Part model, mm, in its own coordinate system. Face numbers are marked on the shaded views. A direction names the side the tool comes from. Give positions to 0.01 mm unless a question says otherwise; leave off trailing zeros. Write each loop counter-clockwise with the first axis right and the second up, starting at its lowest first coordinate (ties: lowest second). Pieces come first, ordered by that corner, then holes.
Autodesk Inventor part; units mm, degrees
ref_plane "Work Plane2" through (2.8, 0, 0) normal (0, 1, 0) x (1, 0, 0)
ref_plane "YZ Plane" through (0, 0, 0) normal (1, 0, 0) x (0, 1, 0)
ref_plane "XZ Plane" through (0, 0, 0) normal (0, 1, 0) x (-1, 0, 0)
sketch "Sketch1" plane through (0, 0, 0) normal (0, 0, 1) x (1, 0, 0)
  line L0 (5.7, 0) -> (45, 0)
  line L1 (45, 0) -> (45, 4.75)
  line L2 (45, 4.75) -> (5.25, 4.75)
  line L3 (0.85, 9.15) -> (0, 9.15)
  line L4 (-9, 0) -> (54, 0)
  line L5 (0, -1.83) -> (0, 10.98)
  line L6 (0, 5) -> (4.1386, 2.9366)
  line L7 (4.1386, 2.9366) -> (5.7, 0)
  line L8 (5.25, 4.75) -> (0.85, 9.15)
  line L9 (0, 9.15) -> (0, 5)
  dimension "d2" = 9.5
  dimension "d3" = 18.3
  dimension "d4" = 5.7
  dimension "d5" = 10
  dimension "d6" = 26.5
  dimension "d7" = 62
  dimension "d13" = 45
  dimension "d14" = 5.25
  dimension "d15" = 45
revolve "Body" add sketch "Sketch1" angle 360 about axis through (5.7, 0, 0) along (1, 0, 0) contours L7 L6 L5 L3 L8 L2 L1 L0
sketch "Sketch2" plane through (0, 0, 0) normal (-1, 0, 0) x (0, 0, 1)
  line L0 (0, -12.81) -> (0, 12.81)
  line L1 (-12.81, 0) -> (12.81, 0)
  line L2 (0, 5) -> (0, 0) construction
  line L3 (0, 0) -> (5, 0) construction
  arc A0 (1.5, 0) -> (0, 1.5) centre (0, 0) ccw construction
  line L4 (0, 0) -> (6.47, 6.47) construction
  arc A1 (1.75, 0) -> (0, 1.75) centre (0, 0) ccw construction
  line L5 (0.595, 4.9645) -> (0.8448, 1.5326)
  line L6 (4.9645, 0.595) -> (1.5326, 0.8448)
  arc A2 (0.8448, 1.5326) -> (1.5326, 0.8448) centre (1.5866, 1.5866) ccw
  arc A3 (5, 0) -> (4.9645, 0.595) centre (0, 0) ccw
  arc A4 (0.595, 4.9645) -> (0, 5) centre (0, 0) ccw
  arc A5 (4.9645, 0.595) -> (0.595, 4.9645) centre (0, 0) ccw
  line L7 (0.595, -4.9645) -> (0.8448, -1.5326)
  line L8 (4.9645, -0.595) -> (1.5326, -0.8448)
  arc A6 (1.5326, -0.8448) -> (0.8448, -1.5326) centre (1.5866, -1.5866) ccw
  arc A7 (4.9645, -0.595) -> (5, 0) centre (0, 0) ccw
  arc A8 (0, -5) -> (0.595, -4.9645) centre (0, 0) ccw
  arc A9 (0.595, -4.9645) -> (4.9645, -0.595) centre (0, 0) ccw
  line L9 (-0.595, 4.9645) -> (-0.8448, 1.5326)
  line L10 (-4.9645, 0.595) -> (-1.5326, 0.8448)
  arc A10 (-1.5326, 0.8448) -> (-0.8448, 1.5326) centre (-1.5866, 1.5866) ccw
  arc A11 (-4.9645, 0.595) -> (-5, 0) centre (0, 0) ccw
  arc A12 (0, 5) -> (-0.595, 4.9645) centre (0, 0) ccw
  arc A13 (-0.595, 4.9645) -> (-4.9645, 0.595) centre (0, 0) ccw
  arc A14 (-4.9645, -0.595) -> (-0.595, -4.9645) centre (0, 0) ccw
  arc A15 (-0.595, -4.9645) -> (0, -5) centre (0, 0) ccw
  arc A16 (-5, 0) -> (-4.9645, -0.595) centre (0, 0) ccw
  line L11 (-4.9645, -0.595) -> (-1.5326, -0.8448)
  arc A17 (-0.8448, -1.5326) -> (-1.5326, -0.8448) centre (-1.5866, -1.5866) ccw
  line L12 (-0.595, -4.9645) -> (-0.8448, -1.5326)
  circle A18 centre (0, 0) radius 9.15
  circle A19 centre (0, 0) radius 5
  dimension "d18" = 45
  dimension "d19" = 3
  dimension "d20" = 3.5
  dimension "d21" = 10
  dimension "d22" = 0.595
extrude "Slot" add sketch "Sketch2" against normal up to next draft 1 contours L7 A6 L8 A9 | A14 L11 A17 L12 | A13 L9 A10 L10 | L6 A2 L5 A5
fillet "Fillet1" radius 0.238 4 edges at (0, 5, 0) (0, 0, 5) (0, -5, 0) (0, 0, -5)
thread "Thread"
chamfer "Chamfer1" distance 1.03 distance2 4.2 1 edges at (45, -4.75, 0) measured on face at (45, -1.1851, 1.0499)
ref_plane "Work Plane2" through (2.8, 0, 0) normal (0, 1, 0) x (1, 0, 0)
equation "\"d2\" = NND"
equation "\"d3\" = KOD"
equation "\"d4\" = STI"
equation "\"d5\" = SDM"
equation "\"d13\" = 0.5 * SEWI"
equation "\"d14\" = KOH"
equation "\"d15\" = NLG"
equation "\"d19\" = 0.3 * SDM"
equation "\"d20\" = 0.35 * SDM"
equation "\"d21\" = SDM"
equation "\"d22\" = 0.5 * SBR"
equation "\"d45\" = STI"
equation "\"d25\" = 0.2 * SBR"
equation "\"d9\" = GEL"
equation "\"d11\" = -0.5 * GD2 + 0.5 * NND"
equation "\"d12\" = SPTZ"
equation "\"NND\" = 9.5"
equation "\"NLG\" = 45"
equation "\"GEL\" = 39.75"
equation "\"KOD\" = 18.3"
equation "\"KOH\" = 5.25"
equation "\"SDM\" = 10"
equation "\"STI\" = 5.7"
equation "\"SBR\" = 1.19"
equation "\"SPTZ\" = 4.2"
equation "\"GD2\" = 7.44"
equation "\"SEWI\" = 90deg"
equation "\"d0\" = NLG"
equation "\"d1\" = KOH"
equation "\"THREADDIA\" = 9.5"
equation "\"TOA\" = 30deg"
equation "\"PTC\" = 2.1"
equation "\"GD1\" = 7.85"
properties part number "ISO 7050 - ST 9.5 x 45 - F - H" material "Steel"
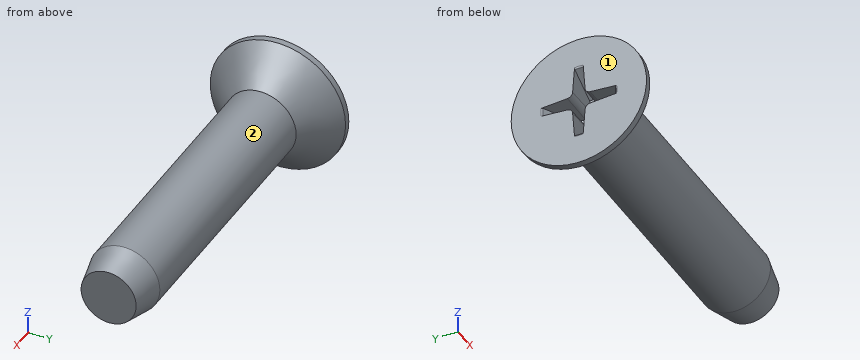
1) Saw through at A-A (x = 9). Write the cut outline in (y, z), and give its area (3 significant figures).
Check result:
outline: circle Ø9.5 at (0, 0)
area: 70.9 mm2
2) Flat gauge pins, fed straight in: P1, Ø1.5, axis at x = 39, z = -3, coming from the +Y side; P2, Ø2, axis at x = 6, z = -1.5, coming from the -Y side; P3, Ø10, axis at x = 40, y = 7, coming from the +Z side. Where does each tip first touch, or does it go through?
Check result:
P1: stops at y = 4.18
P2: stops at y = -4.81
P3: stops at z = 4.31
3) Drill centre lines: L1, parallel to Z at x = 19, y = -0.25; L2, parallel to X at y = -4.5, z = 2.5; L3, parallel to X at y = 5.75, z = -7. Where is each one in solid material? Low to high.
Check result:
L1: z = -4.74 to 4.74
L2: x = 0 to 4.85
L3: x = 0 to 0.94
4) 3-axis set-ups, long thin cutter, end or side, ignore diameter. For the marked faces 1 and 2: which of +Z, -Z, +X, -X, +Y, -Y reach the whole face in a straight line?
Check result:
face 1: +Z, -Z, -X, +Y, -Y
face 2: +X
